Here's how the part is built. I have some questions about the finished solid (model axes, mm). A direction names the side the tool comes from. Round coordinates to 2 decimals unless told otherwise and drop trailing zeros. Loops run counter-clockwise (first coordinate to the right, second up) from the corner with the lowest first, then second, coordinate; pieces in that order, holes last. Notation, with made-up numbers: M -7.5,33 L 15.5,33 A24 cw 15.5,52 Z; hole C 4,0 d10. An arc over 180 degrees is marked long. Answer as a JSON object with one key per item and string values.
from build123d import *

# Parameters (mm, degrees)
SKETCH1_R           = 4.05
SKETCH1_R_2         = 2.5
BOSS_EXTRUDE1_DEPTH = 9
BOSS_EXTRUDE2_START = -1
SKETCH2_R           = 5.25
SKETCH2_R_2         = 2.5
BOSS_EXTRUDE2_DEPTH = 1
SKETCH3_R           = 3.5
SKETCH3_R_2         = 3.1
CUT_EXTRUDE1_DEPTH  = 4.5


with BuildPart() as part:
    # Sketch1 → Boss-Extrude1 (new body)
    with BuildSketch(Plane(origin=(0, 0, 0), x_dir=(1, 0, 0), z_dir=(0, 1, 0))):
        with Locations(Location((0, 0, 0), (0, 0, 270))):
            Circle(SKETCH1_R)
        with Locations(Location((0, 0, 0), (0, 0, 270))):
            Circle(SKETCH1_R_2, mode=Mode.SUBTRACT)
    extrude(amount=BOSS_EXTRUDE1_DEPTH)

    # Sketch2 → Boss-Extrude2 (add)
    with BuildSketch(Plane(origin=(0, 9, 0), x_dir=(1, 0, 0), z_dir=(0, 1, 0)).offset(BOSS_EXTRUDE2_START)):
        with Locations(Location((0, 0, 0), (0, 0, 270))):
            Circle(SKETCH2_R)
        with Locations(Location((0, 0, 0), (0, 0, 270))):
            Circle(SKETCH2_R_2, mode=Mode.SUBTRACT)
    extrude(amount=BOSS_EXTRUDE2_DEPTH)

    # Sketch3 → Cut-Extrude1 (cut)
    with BuildSketch(Plane.XZ):
        with Locations(Location((0, 0, 0), (0, 0, 270))):
            Circle(SKETCH3_R)
        with Locations(Location((0, 0, 0), (0, 0, 270))):
            Circle(SKETCH3_R_2, mode=Mode.SUBTRACT)
    extrude(amount=-CUT_EXTRUDE1_DEPTH, mode=Mode.SUBTRACT)


solid = part.part
Item 1: On a 3-axis mill with a long thin cutter (end or side, diameter ignored), from which of +Z, -Z, +X, -X, +Y, -Y can I reach the whole of each face in a straight line? I mean faces 1 (the face through (-2.44, 4.44, -0.54)), 2 (the face through (0.931, 2.218, -2.957)). Say none if no direction works.
Resolved:
{"face 1": "+Y, -Y", "face 2": "-Y"}
Item 2: I want a section at A-A, the plane x = 0. Please give me the cut outline in (y, z), then the cut area to 3 significant figures.
Resolved:
{"outline": "M 0,-4.05 L 8,-4.05 L 8,-5.25 L 9,-5.25 L 9,-2.5 L 0,-2.5 L 0,-3.1 L 4.5,-3.1 L 4.5,-3.5 L 0,-3.5 Z; M 0,2.5 L 9,2.5 L 9,5.25 L 8,5.25 L 8,4.05 L 0,4.05 L 0,3.5 L 4.5,3.5 L 4.5,3.1 L 0,3.1 Z", "area": "26.7 mm²"}
Item 3: I want a section at D-D, the plane y = 6.5. Please give me the cut outline in (x, z), then the cut area to 3 significant figures.
Resolved:
{"outline": "C 0,0 d8.1; hole C 0,0 d5", "area": "31.9 mm²"}
Item 4: I want a section at B-B, the plane z = 0. Please give me the cut outline in (x, y), then the cut area to 3 significant figures.
Resolved:
{"outline": "M -5.25,8 L -4.05,8 L -4.05,0 L -3.5,0 L -3.5,4.5 L -3.1,4.5 L -3.1,0 L -2.5,0 L -2.5,9 L -5.25,9 Z; M 2.5,0 L 3.1,0 L 3.1,4.5 L 3.5,4.5 L 3.5,0 L 4.05,0 L 4.05,8 L 5.25,8 L 5.25,9 L 2.5,9 Z", "area": "26.7 mm²"}
Item 5: I want a section at C-C, the plane y = 1.5. Please give me the cut outline in (x, z), then the cut area to 3 significant figures.
Resolved:
{"outline": "C 0,0 d8.1; C 0,0 d6.2; hole C 0,0 d7; hole C 0,0 d5", "area": "23.6 mm²"}
Item 6: Please list where these lines run through material, in increasing order: probe 1 along X at (y, z) = (1.15, 0); probe 2 along X at (y, z) = (3.75, -1.5); probe 3 along X at (y, z) = (6, 0). Write a range as from..to.
Resolved:
{"probe 1": "-4.05..-3.5, -3.1..-2.5, 2.5..3.1, 3.5..4.05", "probe 2": "-3.76..-3.16, -2.71..-2, 2..2.71, 3.16..3.76", "probe 3": "-4.05..-2.5, 2.5..4.05"}
Item 7: If we mould it in two halves opening along X, with no side actions, what happens to faces 3 (the face through (-3, 8, 3)), 4 (the face through (-3.593, 3.944, 1.869)), 5 (the face through (-3.417, 2.218, 0.759))? For each: pulls with the +X half, pulls with the -X half, needs draft (parallel to the pull), parting line crosses it, or undercut.
Resolved:
{"face 3": "needs draft", "face 4": "parting line crosses it", "face 5": "undercut"}
Item 8: I'm going to push flat-ended pins straight in: pin 1 Ø1 at (x, y) = (0, 5.5) entering from -Z; pin 2 Ø2 at (y, z) = (5.5, 0) entering from -X; pin 3 Ø2 at (x, y) = (-3.5, 1) entering from -Z. Where does each tip first touch, or does it pass through?
Resolved:
{"pin 1": "z = -4.05", "pin 2": "x = -4.05", "pin 3": "z = -3.19"}
